Part model, mm, in its own coordinate system. A direction names the side the tool comes from. Round coordinates to 2 decimals unless told otherwise and drop trailing zeros. Write each loop counter-clockwise with the first axis right and the second up, starting at its lowest first coordinate (ties: lowest second). Pieces come first, ordered by that corner, then holes. Notation, with made-up numbers: M 16.25,-9.5 L 74.25,-9.5 A8 ccw 74.25,-5.5 Z; hole C 35.25,-15 d6. An arc over 180 degrees is marked long. Use a Markdown table: item, result. Add a question column.
1) Which spindle directions (+Z, -Z, +X, -X, +Y, -Y) get a long thin tool onto all of the face, cutting with end or side? Do faces 1 (the face through (-17, 2, -12.8)), 2 (the face through (-3, 3, -6.8)), 3 (the face through (-11.4, 2, -5)), 4 (the face through (1, 1.5, -41)). Say none if no direction does.
2) Drop flat-ended pins along their axis: P1, Ø1, axis at x = -22.5, z = -54, coming from the +Y side; P2, Ø1.5, axis at x = -4, y = 2, coming from the -Z side; P3, Ø1.5, axis at x = 0.5, z = -41.5, coming from the -Y side; P4, Ø12, axis at x = -6.5, z = -52.5, coming from the +Y side. Give the stop position or say it passes through.
3) Two-plate mould, pull along Z, no slides. Class faces 5 (the face through (-1, 3, -37.45)), 6 (the face through (-0.86, 0.76, -64.1)), 7 (the face through (-17, 2, 2.6)): released by +Z, released by -Z, zero draft, split by the parting line, or undercut.
4) Slice it at B-B on z = -6. Write the cut outline in (x, y), plus the area to 4 significant figures.
5) Wall check: probe 1 along X at (y, z) = (1.1, -21); probe 2 along Z at (x, y) = (-26.5, 1.05) (3 decimals); probe 3 along Z at (x, y) = (-2, 3.1). Give the ranges that are in metal, low to high.
6) Slice it at C-C on x = -1.5. Write the cut outline in (y, z).
7) Slice it at A-A on x = -10. Write the cut outline in (y, z).
8) Slice it at D-D on x = -16. Write the cut outline in (y, z), plus the area to 3 significant figures.
Autodesk Inventor part; units mm, degrees
ref_plane "YZ Plane" through (0, 0, 0) normal (1, 0, 0) x (0, 1, 0)
ref_plane "XZ Plane" through (0, 0, 0) normal (0, 1, 0) x (-1, 0, 0)
ref_plane "XY Plane" through (0, 0, 0) normal (0, 0, 1) x (1, 0, 0)
sketch "Sketch1" plane through (0, 0, 0) normal (0, 1, 0) x (-1, 0, 0)
  line L0 (0, 0) -> (30, 0)
  line L1 (30, 0) -> (30, -65)
  line L2 (30, -65) -> (0, -65)
  line L3 (0, -65) -> (0, 0)
  circle A0 centre (26.5, -3.5) radius 1.375
  circle A1 centre (3.5, -3.5) radius 1.375
  circle A2 centre (26.5, -61.5) radius 1.375
  circle A3 centre (3.5, -61.5) radius 1.375
  line L4 (15, 0) -> (15, -65)
  line L5 (30, -32.5) -> (0, -32.5)
  dimension "d0" = 65
  dimension "d1" = 30
  dimension "d2" = 3.5
  dimension "d3" = 3.5
  dimension "d4" = 3.5
  dimension "d5" = 3.5
  dimension "d6" = 3.5
  dimension "d7" = 3.5
  dimension "d8" = 3.5
  dimension "d9" = 3.5
  dimension "d10" = 2.75
  dimension "d11" = 2.75
  dimension "d12" = 2.75
  dimension "d13" = 2.75
  dimension "d14" = 15
  dimension "d15" = 32.5
extrude "Extrusion1" add sketch "Sketch1" along normal blind 1.5
fillet "Fillet1" radius 3 4 edges at (-30, 0.75, 0) (0, 0.75, 0) (0, 0.75, -65) (-30, 0.75, -65)
sketch "Sketch2" plane through (0, 1.5, 0) normal (0, 1, 0) x (1, 0, 0)
  line L0 (-6.9, 6.8) -> (0.6, 6.8)
  line L1 (0.6, 6.8) -> (0.6, 18)
  line L2 (0.6, 18) -> (-6.9, 18)
  line L3 (-6.9, 18) -> (-6.9, 6.8)
  line L4 (-27, 0) -> (-3, 0)
  line L5 (-15, 0) -> (-15, 64.9233)
  line L6 (-30, 62) -> (-30, 3)
  line L7 (0.6, 12.4) -> (-6.9, 12.4)
  line L8 (-4.1, 57.95) -> (1.4, 57.95)
  line L9 (1.4, 57.95) -> (1.4, 50.05)
  line L10 (1.4, 50.05) -> (-4.1, 50.05)
  line L11 (-4.1, 50.05) -> (-4.1, 57.95)
  line L12 (-4.1, 45.35) -> (1.4, 45.35)
  line L13 (1.4, 45.35) -> (1.4, 37.45)
  line L14 (1.4, 37.45) -> (-4.1, 37.45)
  line L15 (-4.1, 37.45) -> (-4.1, 45.35)
  line L16 (-4.1, 41.4) -> (1.4, 41.4)
  line L17 (-4.1, 54) -> (1.4, 54)
  line L18 (-22.4, 12.8) -> (-11.4, 12.8)
  line L19 (-11.4, 12.8) -> (-11.4, -2.6)
  line L20 (-11.4, -2.6) -> (-22.4, -2.6)
  line L21 (-22.4, -2.6) -> (-22.4, 12.8)
  line L22 (-16.9, 12.8) -> (-16.9, -2.6)
  line L23 (0, 3) -> (0, 62)
  line L24 (-23.5, 65.9) -> (-6.5, 65.9)
  line L25 (-6.5, 65.9) -> (-6.5, 61.9)
  line L26 (-6.5, 61.9) -> (-23.5, 61.9)
  line L27 (-23.5, 61.9) -> (-23.5, 65.9)
  line L28 (-15, 65.9) -> (-15, 61.9)
  point P0 (0, 0)
  dimension "d19" = 11.2
  dimension "d20" = 7.5
  dimension "d21" = 15
  dimension "d23" = 12.4
  dimension "d24" = 7.9
  dimension "d25" = 7.9
  dimension "d26" = 5.5
  dimension "d27" = 3.95
  dimension "d28" = 3.95
  dimension "d29" = 41.4
  dimension "d30" = 54
  dimension "d32" = 30.6
  dimension "d33" = 31.4
  dimension "d34" = 11
  dimension "d35" = 15.4
  dimension "d36" = 2.6
  dimension "d37" = 5.5
  dimension "d38" = 16.9
  dimension "d39" = 65.9
  dimension "d40" = 4
  dimension "d41" = 17
  dimension "d42" = 8.5
  dimension "d43" = 15
extrude "Extrusion2" add sketch "Sketch2" along normal blind 3.25 contours L3 L7 L23 L0 | L23 L7 L1 L0 | L3 L2 L23 L7 | L23 L2 L1 L7
extrude "Extrusion3" add sketch "Sketch2" along normal blind 2.55 contours L10 L11 L17 L23 | L23 L17 L9 L10 | L14 L15 L16 L23 | L23 L16 L13 L14 | L23 L12 L13 L16 | L16 L15 L12 L23 | L23 L8 L9 L17 | L17 L11 L8 L23
extrude "Extrusion4" add sketch "Sketch2" along normal blind 1.25 contours L26 L27 L24 L28 L5 | L5 L28 L24 L25 L26
extrude "Extrusion5" add sketch "Sketch2" along normal blind 1.35 contours L21 L18 L22 L4 | L4 L22 L20 L21 | L22 L18 L5 L4 | L4 L19 L20 L22 | L5 L18 L19 L4
chamfer "Chamfer1" distance 1.1735 angle 45 2 edges at (0.3, 1.5, -6.8) (0.3, 1.5, -18)
chamfer "Chamfer2" distance 0.889 angle 45 4 edges at (0.7, 1.5, -37.45) (0.7, 1.5, -45.35) (0.7, 1.5, -50.05) (0.7, 1.5, -57.95)
sketch "Sketch4" plane through (0, 1.5, 0) normal (0, 1, 0) x (1, 0, 0)
  line L0 (-28.85, 7.05) -> (-23.35, 7.05) construction
  line L1 (-23.35, 7.05) -> (-23.35, 57.95) construction
  line L2 (-23.35, 57.95) -> (-28.85, 57.95) construction
  line L3 (-28.85, 57.95) -> (-28.85, 7.05) construction
  line L4 (-30, 62) -> (-30, 3) construction
  line L5 (-27, 0) -> (-22.4, 0) construction
  line L6 (-23.5, 65) -> (-27, 65) construction
  line L7 (-27.37, 8.37) -> (-28.85, 8.37) construction
  line L8 (-24.83, 8.37) -> (-23.35, 8.37) construction
  line L9 (-27.37, 8.37) -> (-27.37, 7.05) construction
  line L10 (-27.37, 56.63) -> (-27.37, 57.95) construction
  line L11 (-24.83, 8.37) -> (-24.83, 7.05) construction
  line L12 (-24.83, 56.63) -> (-24.83, 57.95) construction
  circle A0 centre (-27.37, 8.37) radius 0.508
  circle A1 centre (-27.37, 10.91) radius 0.508
  circle A2 centre (-27.37, 13.45) radius 0.508
  circle A3 centre (-27.37, 15.99) radius 0.508
  circle A4 centre (-27.37, 18.53) radius 0.508
  circle A5 centre (-27.37, 21.07) radius 0.508
  circle A6 centre (-27.37, 23.61) radius 0.508
  circle A7 centre (-27.37, 26.15) radius 0.508
  circle A8 centre (-27.37, 28.69) radius 0.508
  circle A9 centre (-27.37, 31.23) radius 0.508
  circle A10 centre (-27.37, 33.77) radius 0.508
  circle A11 centre (-27.37, 36.31) radius 0.508
  circle A12 centre (-27.37, 38.85) radius 0.508
  circle A13 centre (-27.37, 41.39) radius 0.508
  circle A14 centre (-27.37, 43.93) radius 0.508
  circle A15 centre (-27.37, 46.47) radius 0.508
  circle A16 centre (-27.37, 49.01) radius 0.508
  circle A17 centre (-27.37, 51.55) radius 0.508
  circle A18 centre (-27.37, 54.09) radius 0.508
  circle A19 centre (-27.37, 56.63) radius 0.508
  circle A20 centre (-24.83, 8.37) radius 0.508
  circle A21 centre (-24.83, 10.91) radius 0.508
  circle A22 centre (-24.83, 13.45) radius 0.508
  circle A23 centre (-24.83, 15.99) radius 0.508
  circle A24 centre (-24.83, 18.53) radius 0.508
  circle A25 centre (-24.83, 21.07) radius 0.508
  circle A26 centre (-24.83, 23.61) radius 0.508
  circle A27 centre (-24.83, 26.15) radius 0.508
  circle A28 centre (-24.83, 28.69) radius 0.508
  circle A29 centre (-24.83, 31.23) radius 0.508
  circle A30 centre (-24.83, 33.77) radius 0.508
  circle A31 centre (-24.83, 36.31) radius 0.508
  circle A32 centre (-24.83, 38.85) radius 0.508
  circle A33 centre (-24.83, 41.39) radius 0.508
  circle A34 centre (-24.83, 43.93) radius 0.508
  circle A35 centre (-24.83, 46.47) radius 0.508
  circle A36 centre (-24.83, 49.01) radius 0.508
  circle A37 centre (-24.83, 51.55) radius 0.508
  circle A38 centre (-24.83, 54.09) radius 0.508
  circle A39 centre (-24.83, 56.63) radius 0.508
  point P0 (0, 0)
  point P1 (-27.37, 21.07)
  point P2 (-27.37, 26.15)
  point P3 (-27.37, 31.23)
  point P4 (-27.37, 36.31)
  point P5 (-27.37, 51.55)
  point P6 (-24.83, 21.07)
  point P7 (-24.83, 26.15)
  point P8 (-24.83, 31.23)
  point P9 (-24.83, 36.31)
  point P10 (-24.83, 51.55)
  dimension "d63" = 1.15
  dimension "d64" = 50.9
  dimension "d65" = 7.05
  dimension "d66" = 7.05
  dimension "d67" = 5.5
  dimension "d68" = 2.54
  dimension "d71" = 2.54
  dimension "d74" = 2.54
  dimension "d77" = 1.016
  dimension "d80" = 2.54
  dimension "d83" = 2.54
extrude "Extrusion7" cut sketch "Sketch4" against normal through all
equation "\"d11\" = d10"
equation "\"d12\" = d10"
equation "\"d13\" = d10"
equation "\"d14\" = 0.5 * d1"
equation "\"d15\" = 0.5 * d0"
equation "\"d21\" = d14"
equation "\"d25\" = d24"
equation "\"d27\" = 0.5 * d25"
equation "\"d37\" = 0.5 * d34"
equation "\"d42\" = 0.5 * d41"
equation "\"d43\" = d14"
equation "\"d65\" = d66"
properties part number "pizero_model no gpio" material "UHMW, Black"
Entries:
| question | item | result |
|---|---|---|
| 1 | face 1 | -X, +Y |
| 1 | face 2 | +Z, +X, +Y |
| 1 | face 3 | +Z, +Y |
| 1 | face 4 | +Z, -Z, +X, -Y |
| 2 | P1 | stops at y = 1.5 |
| 2 | P2 | stops at z = -65 |
| 2 | P3 | stops at y = 0 |
| 2 | P4 | stops at y = 4.05 |
| 3 | face 5 | undercut |
| 3 | face 6 | released by -Z |
| 3 | face 7 | released by +Z |
| 4 | outline | M -30,0 L 0,0 L 0,1.5 L -11.4,1.5 L -11.4,2.85 L -22.4,2.85 L -22.4,1.5 L -30,1.5 Z |
| 4 | area | 59.85 mm^2 |
| 5 | probe 1 | x = -30 to -27.87, -26.87 to -25.33, -24.33 to 0 |
| 5 | probe 2 | z = -65 to -62.875, -60.125 to -4.875, -2.125 to 0 |
| 5 | probe 3 | z = -57.95 to -50.05, -45.35 to -37.45, -18 to -6.8 |
| 6 | outline | M 0,-64.6 L 1.5,-64.6 L 1.5,-57.95 L 4.05,-57.95 L 4.05,-50.05 L 1.5,-50.05 L 1.5,-45.35 L 4.05,-45.35 L 4.05,-37.45 L 1.5,-37.45 L 1.5,-18 L 4.75,-18 L 4.75,-6.8 L 1.5,-6.8 L 1.5,-0.4 L 0,-0.4 Z |
| 7 | outline | M 0,-65 L 1.5,-65 L 1.5,-65.9 L 2.75,-65.9 L 2.75,-61.9 L 1.5,-61.9 L 1.5,0 L 0,0 Z |
| 8 | outline | M 0,-65 L 1.5,-65 L 1.5,-65.9 L 2.75,-65.9 L 2.75,-61.9 L 1.5,-61.9 L 1.5,-12.8 L 2.85,-12.8 L 2.85,2.6 L 1.5,2.6 L 1.5,0 L 0,0 Z |
| 8 | area | 123 mm^2 |
